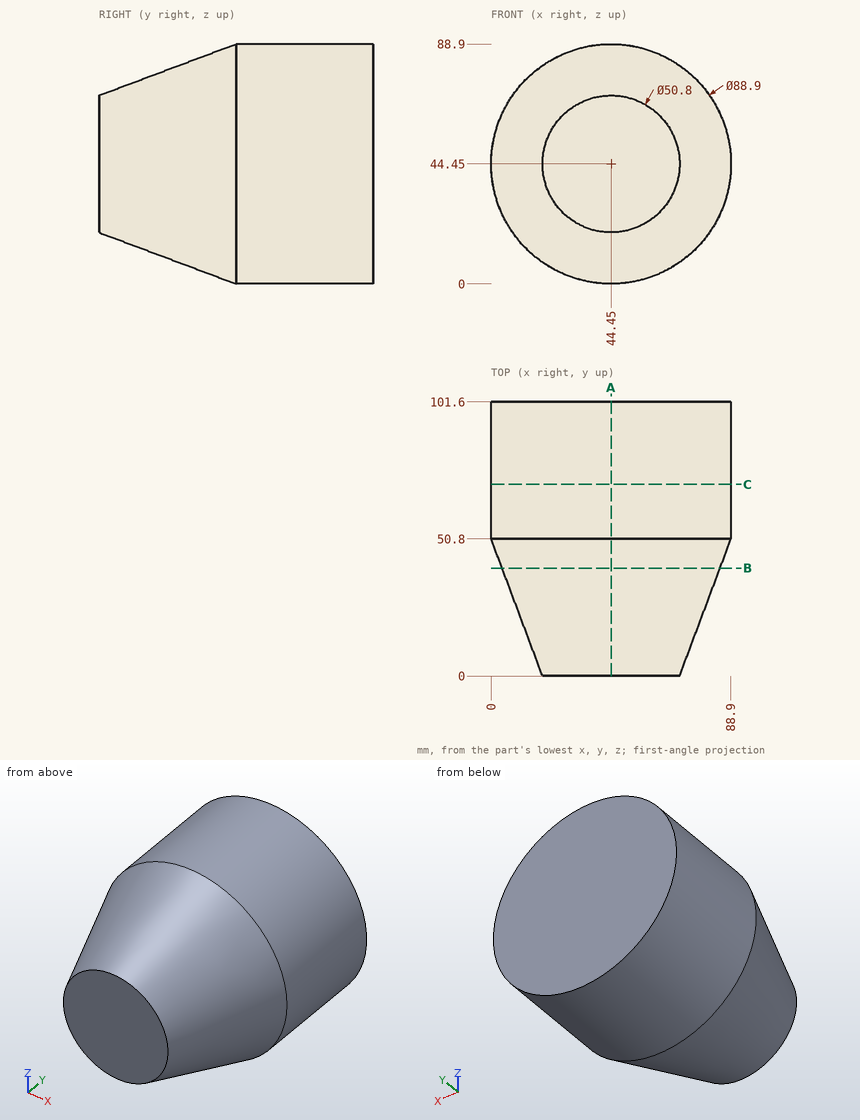
Design review of the part shown in the three views and the two pictorial views. Dimensions are in mm from the part's minimum x, y and z. Round coordinates to 2 decimals unless told otherwise and drop trailing zeros. Write each loop counter-clockwise with the first axis right and the second up, starting at its lowest first coordinate (ties: lowest second). Pieces come first, ordered by that corner, then holes. Notation, with made-up numbers: (10, 31.25) - (39, 31.25) arc R36 cw to (39, 66.25) - close; hole circle Ø7 at (25.25, 84.25). An arc over 180 degrees is marked (long way). Return JSON: item names as keys, results as strings. Group by question number.
Item 1: We need section C-C on y = 71. Write out the cut boundary in (x, z).
Item 2: Insertion check: P1, Ø3, axis at x = 13, y = 21, coming from the -Z side; P2, Ø2, axis at y = 85.5, z = 56.5, coming from the +X side; P3, Ø12, axis at y = 19, z = 58, coming from the +X side. Each pin has a flat end and moves straight along its axis. Give the tip position at first contact, or say it passes through.
Item 3: We need section A-A on x = 44.45. Write out the cut boundary in (y, z), and give its area (3 significant figures).
Item 4: We need section B-B on y = 40. Write out the cut boundary in (x, z).
Item 5: For probe 1 along Y at (x, z) = (60, 16.5); probe 2 along Y at (x, z) = (78.5, 27); probe 3 along Z at (x, y) = (48, 18.5), list the stretches that pass through material, from the lowest coordinate up. Write a range as [from, to].
Model answer:
{
 "1": {"outline": "circle Ø88.9 at (44.45, 44.45)"},
 "2": {"P1": "stops at z = 29.69", "P2": "stops at x = 87.5", "P3": "stops at x = 77.3"},
 "3": {"outline": "(0, 19.05) - (50.8, 0) - (101.6, 0) - (101.6, 88.9) - (50.8, 88.9) - (0, 69.85) - close", "area": "8,060 mm²"},
 "4": {"outline": "circle Ø80.8 at (44.45, 44.45)"},
 "5": {"probe 1": "y = [17.56, 101.6]", "probe 2": "y = [34.3, 101.6]", "probe 3": "z = [12.31, 76.59]"}
}
